Geometry: see drawing. Coordinates: mm, zero at the bounding-box minimum. Give positions to 0.01 mm unless a question says otherwise; leave off trailing zeros. Write each loop counter-clockwise with the first axis right and the second up, starting at its lowest first coordinate (ties: lowest second). Pieces come first, ordered by that corner, then holes. Notation, with made-up numbers: M -21.5,-4.75 L 28.5,-4.75 A24 cw 28.5,11.25 Z; hole C 18,49.25 d4. An arc over 180 degrees is marked long. Use a Markdown table: item, result. Add a question column.
1) Pin query (flat end, axial travel): pin 1 (2.5 mm diameter, centred on y = 9.1, z = 90, fed in from +X); pin 2 (1.8 mm diameter, centred on x = 2, y = 64.5, fed in from -Z). Return the tip coordinate at first contact, or that it passes through.
2) Section A-A on y = 65.3. State how many separate pieces and enclosed holes the cut face has.
3) Section B-B on z = 90. Return the cut outline in (x, y).
4) Section C-C on y = 9.1. Return the cut outline in (x, z).
5) Line query: line 1 (Y direction, x = 5.8, z = 141.5); line 2 (Z direction, x = 1.4, y = 63.5); line 3 (Y direction, x = 4.35, z = 90). Output: solid intervals per line, ascending.
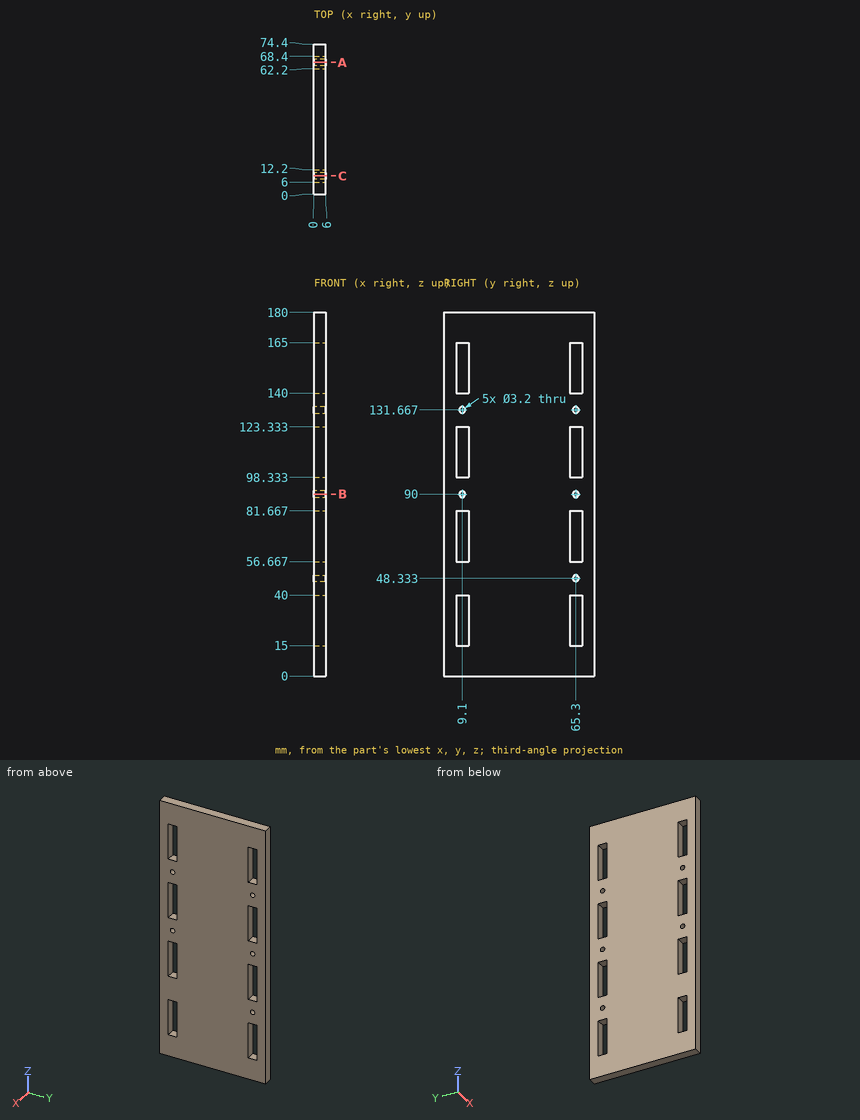
Found:
| question | item | result |
|---|---|---|
| 1 | pin 1 | through |
| 1 | pin 2 | z = 0 |
| 2 | separate pieces | 8 |
| 2 | enclosed holes | 0 |
| 3 | outline | M 0,0 L 6,0 L 6,7.5 L 0,7.5 Z; M 0,10.7 L 6,10.7 L 6,63.7 L 0,63.7 Z; M 0,66.9 L 6,66.9 L 6,74.4 L 0,74.4 Z |
| 4 | outline | M 0,0 L 6,0 L 6,15 L 0,15 Z; M 0,40 L 6,40 L 6,56.67 L 0,56.67 Z; M 0,81.67 L 6,81.67 L 6,88.4 L 0,88.4 Z; M 0,91.6 L 6,91.6 L 6,98.33 L 0,98.33 Z; M 0,123.33 L 6,123.33 L 6,130.07 L 0,130.07 Z; M 0,133.27 L 6,133.27 L 6,140 L 0,140 Z; M 0,165 L 6,165 L 6,180 L 0,180 Z |
| 5 | line 1 | 0 to 6, 12.2 to 62.2, 68.4 to 74.4 |
| 5 | line 2 | 0 to 15, 40 to 56.67, 81.67 to 98.33, 123.33 to 140, 165 to 180 |
| 5 | line 3 | 0 to 7.5, 10.7 to 63.7, 66.9 to 74.4 |
